Can you work these out from the drawing? Everything is in mm from the part's minimum corner. Give positions to 0.01 mm unless a question says otherwise; leave off trailing zeros. Write each loop counter-clockwise with the first axis right and the second up, starting at its lowest first coordinate (ties: lowest second). Pieces come first, ordered by that corner, then holes. Notation, with made-up numbers: M 16,54.25 L 52,54.25 A19 cw 52,61.25 Z; hole C -8.5,-9.5 d7. An arc over 180 degrees is marked long. One line per item, written item: value.
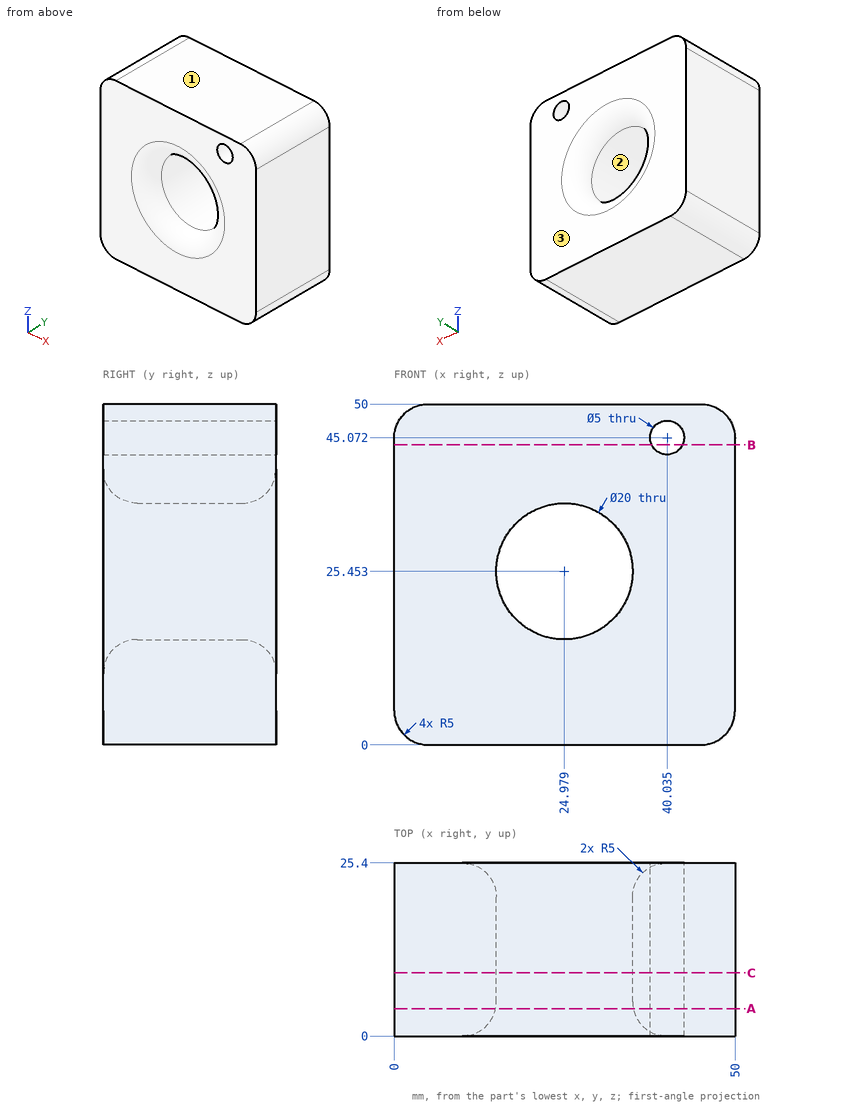
1) I'm going to push a flat-ended pin straight in: pin 1 (6 mm diameter, centred on x = 20, z = 31, fed in from +Y). Where does the tip first touch, or does it pass through?
Outcome:
pin 1: stops at y = 22.48
2) If we section it at B-B, the plane z = 44: Write out the boundary of the cut face in (x, y), then the cut area to 3 significant figures.
Outcome:
outline: M 0,0 L 37.78,0 L 37.78,25.4 L 0,25.4 Z; M 42.29,0 L 50,0 L 50,25.4 L 42.29,25.4 Z
area: 1,160 mm^2
3) We'd pull the mould along Z, two halves only. Please class the marked faces 1, 2 and 3: pulls with the +Z half, pulls with the -Z half, needs draft (parallel to the pull), parting line crosses it, or undercut.
Outcome:
face 1: pulls with the +Z half
face 2: undercut
face 3: needs draft
4) If we section it at A-A, the plane y = 4: Write out the boundary of the cut face in (x, z) (1 decimal).
Outcome:
outline: M 0,5 A5 ccw 5,0 L 45,0 A5 ccw 50,5 L 50,45 A5 ccw 45,50 L 5,50 A5 ccw 0,45 Z; hole C 25,25.5 d20.2; hole C 40,45.1 d5
5) If we section it at C-C, the plane y = 9.25: Write out the boundary of the cut face in (x, z) (1 decimal), then the cut area to 3 significant figures.
Outcome:
outline: M 0,5 A5 ccw 5,0 L 45,0 A5 ccw 50,5 L 50,45 A5 ccw 45,50 L 5,50 A5 ccw 0,45 Z; hole C 25,25.5 d20; hole C 40,45.1 d5
area: 2,140 mm^2
6) Please list where these lines run through material, in increasing order: L1, parallel to Z at x = 31, y = 16.25; L2, parallel to Z at x = 17, y = 4 (1 decimal); L3, parallel to X at y = 13.75, z = 29.5 (1 decimal). Write a range as from..to.
Outcome:
L1: z = 0..17.47, 33.44..50
L2: z = 0..19.3, 31.6..50
L3: x = 0..15.8, 34.1..50
